Answer from the drawing. Dimensions are ordinates in mm from the lowest x, y and z of the part. Round coordinates to 2 decimals unless told otherwise and drop trailing zeros. Write each loop counter-clockwise with the first axis right and the second up, starting at its lowest first coordinate (ties: lowest second). Pieces come first, ordered by that corner, then holes. Notation, with made-up numbers: (-15, 8.25) - (-2, 8.25) arc R26 ccw to (-2, 31.25) - close; hole circle Ø4 at (85, 53.5). An arc over 180 degrees is marked (long way). Use a Markdown table: item, result. Add a question column.
1) A cutting plane is placed at B-B (y = 42). Give the vertices of the cut face in (x, z), then the cut area to 3 significant figures.
2) Find the intervals of material crossed by probe 1 along Z at (x, y) = (27, 25); probe 2 along Z at (x, y) = (22, 12.5), in increasing order. Write a range as from..to.
3) Each of these flat-tipped pins is pushed along its axis until it touches: P1, Ø12, axis at x = 20, y = 39.5, coming from the -Z side; P2, Ø5, axis at x = 34.5, z = 35.5, coming from the +Y side; P3, Ø1.5, axis at x = 2, z = 2, coming from the -Y side. Where does it stop, or does it pass through?
4) Determine the mould class of the marked faces 1, 2 and 3 for opening direction Z: +Z half, -Z half, draft (parallel to the pull), parting line (faces both ways), or undercut.
5) A cutting plane is placed at A-A (z = 25). Give the vertices of the cut face in (x, y), then the cut area to 3 significant figures.
6) A cutting plane is placed at C-C (x = 28.5). Give the vertices of the cut face in (y, z).
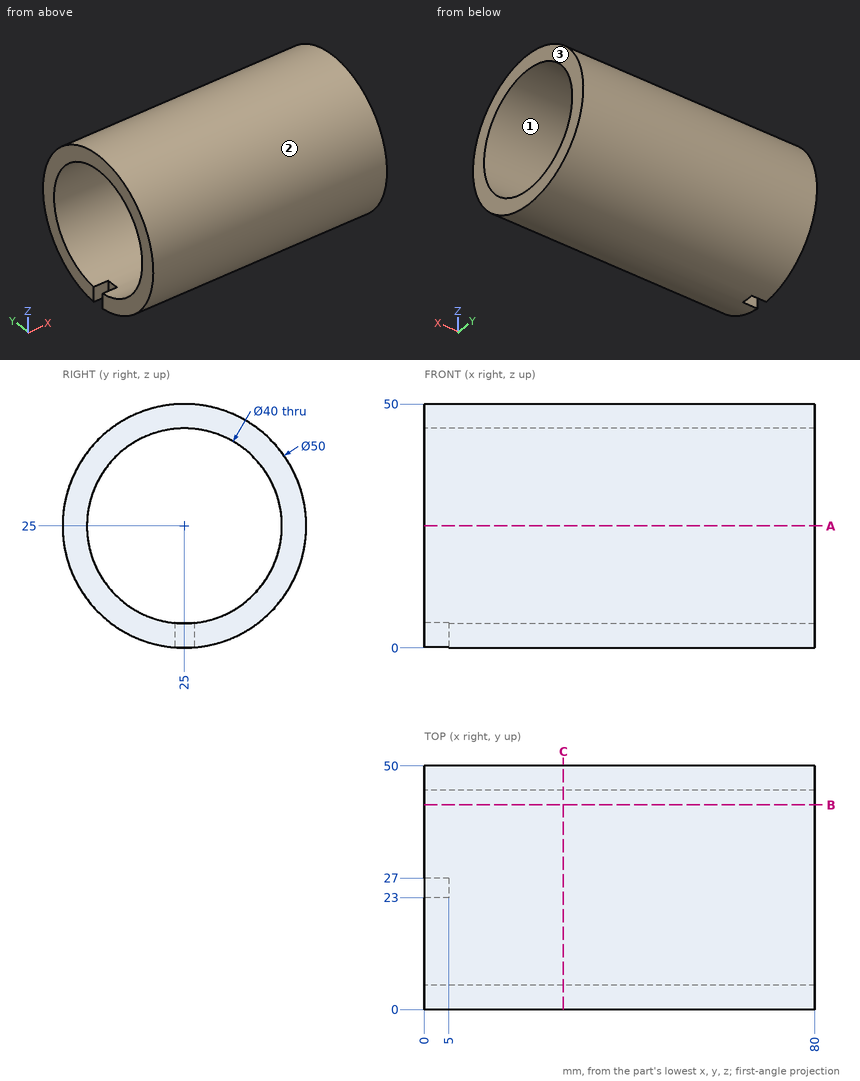
Entries:
| question | item | result |
|---|---|---|
| 1 | outline | (0, 6.67) - (80, 6.67) - (80, 14.46) - (0, 14.46) - close; (0, 35.54) - (80, 35.54) - (80, 43.33) - (0, 43.33) - close |
| 1 | area | 1,250 mm² |
| 2 | probe 1 | z = 0..5, 45..50 |
| 2 | probe 2 | z = 3.35..9.39, 40.61..46.65 |
| 3 | P1 | stops at z = 1.49 |
| 3 | P2 | stops at y = 48.69 |
| 3 | P3 | stops at y = 13.6 |
| 4 | face 1 | undercut |
| 4 | face 2 | parting line |
| 4 | face 3 | draft |
| 5 | outline | (0, 0) - (80, 0) - (80, 5) - (0, 5) - close; (0, 45) - (80, 45) - (80, 50) - (0, 50) - close |
| 5 | area | 800 mm² |
| 6 | outline | circle Ø50 at (25, 25); hole circle Ø40 at (25, 25) |
